from build123d import *

# Parameters (mm, degrees)
F0_R      = 22.5
F1_DEPTH  = 3
F2_R      = 5
F3_DEPTH  = 70
F4_R      = 12
F5_DEPTH  = 28
F6_R      = 6
F7_W      = 19.57
F7_H      = 20
F8_DEPTH  = 12.5
F9_R      = 9
F9_R_2    = 4
F10_DEPTH = 12.5


with BuildPart() as f1:
    # F0 (on Top) → F1 (new body)
    with BuildSketch(Plane.XY):
        Circle(F0_R)
    extrude(amount=F1_DEPTH)

    # F2 (on Top) → F3 (join)
    with BuildSketch(Plane.XY):
        Circle(F2_R)
    extrude(amount=F3_DEPTH)

    # F4 (on face) → F5 (join)
    with BuildSketch(Plane(origin=(0, 0, 0), x_dir=(1, 0, 0), z_dir=(0, 0, -1))):
        Circle(F4_R)
    extrude(amount=F5_DEPTH)

    # F6
    f6_edges = [f1.edges().sort_by_distance(p)[0] for p in [
        (-12, 0, -28),
    ]]
    fillet(f6_edges, radius=F6_R)

    # F7 (on Front) → F8 (cut, symmetric)
    with BuildSketch(Plane.XZ):
        with Locations((17.285, -18)):
            Rectangle(F7_W, F7_H)
        with Locations((-17.285, -18)):
            Rectangle(F7_W, F7_H)
    extrude(amount=F8_DEPTH, both=True, mode=Mode.SUBTRACT)

    # F9 (on Right) → F10 (join, symmetric)
    with BuildSketch(Plane.YZ):
        with Locations((0, -18)):
            Circle(F9_R)
        with Locations((0, -18)):
            Circle(F9_R_2, mode=Mode.SUBTRACT)
    extrude(amount=F10_DEPTH, both=True)


solid = f1.part
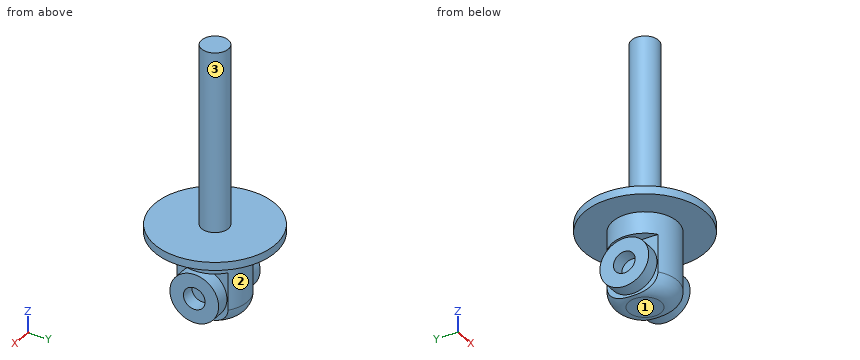
Work out the finished part from the listing and answer in its coordinate system (mm). Face numbers are marked on the shaded views. Round coordinates to 2 decimals unless told otherwise and drop trailing zeros. Write each loop counter-clockwise with the first axis right and the second up, starting at its lowest first coordinate (ties: lowest second). Pieces come first, ordered by that corner, then holes.
1) Straight lines are drawn through the part: line 1 (Z direction, x = 10, y = 0); line 2 (X direction, y = 3, z = 18); line 3 (Y direction, x = 10, z = -13). For each, find the intervals that lie inside material, in ascending order.
2) A cutting plane is placed at A-A (z = -18). Give the vertices of the cut face in (x, y), plus the area to 3 significant figures.
3) The mould has two halves that part along Z. Classify the marked faces 1, 2 and 3: pulls with the +Z half, pulls with the -Z half, needs draft (parallel to the pull), parting line crosses it, or undercut.
4) A cutting plane is placed at C-C (x = -17). Give the vertices of the cut face in (y, z).
5) Given pin 1 Ø5 at (y, z) = (0, -18) entering from -X; pin 2 Ø6.5 at (y, z) = (-1.5, -17.5) entering from +X; pin 3 Ø20 at (y, z) = (-2.5, -14) entering from -X, each flat-ended and moving along its own axis, determine where each tip first touches the part or whether it passes through.
6) A cutting plane is placed at D-D (y = -19). Give the vertices of the cut face in (x, z), plus the area to 3 significant figures.
7) A cutting plane is placed at B-B (z = 13.5). Give the vertices of the cut face in (x, y).
Completed:
1. line 1: z = -27 to -22, -14 to -9, -8 to 3
1. line 2: x = -4 to 4
1. line 3: y = -7.48 to 7.48
2. outline: (-12.5, -9) - (-7.5, -9) - (-7.5, -9.37) arc R12 ccw to (7.5, -9.37) - (7.5, -9) - (12.5, -9) - (12.5, -4) - (7.5, -4) - (7.5, 4) - (12.5, 4) - (12.5, 9) - (7.5, 9) - (7.5, 9.37) arc R12 ccw to (-7.5, 9.37) - (-7.5, 9) - (-12.5, 9) - (-12.5, 4) - (-7.5, 4) - (-7.5, -4) - (-12.5, -4) - close
2. area: 435 mm2
3. face 1: pulls with the -Z half
3. face 2: undercut
3. face 3: needs draft
4. outline: (-14.74, 0) - (14.74, 0) - (14.74, 3) - (-14.74, 3) - close
5. pin 1: stops at x = -7.5
5. pin 2: stops at x = 12.5
5. pin 3: stops at x = -12.5
6. outline: (-12.05, 0) - (12.05, 0) - (12.05, 3) - (-12.05, 3) - close
6. area: 72.3 mm2
7. outline: circle Ø10 at (0, 0)
